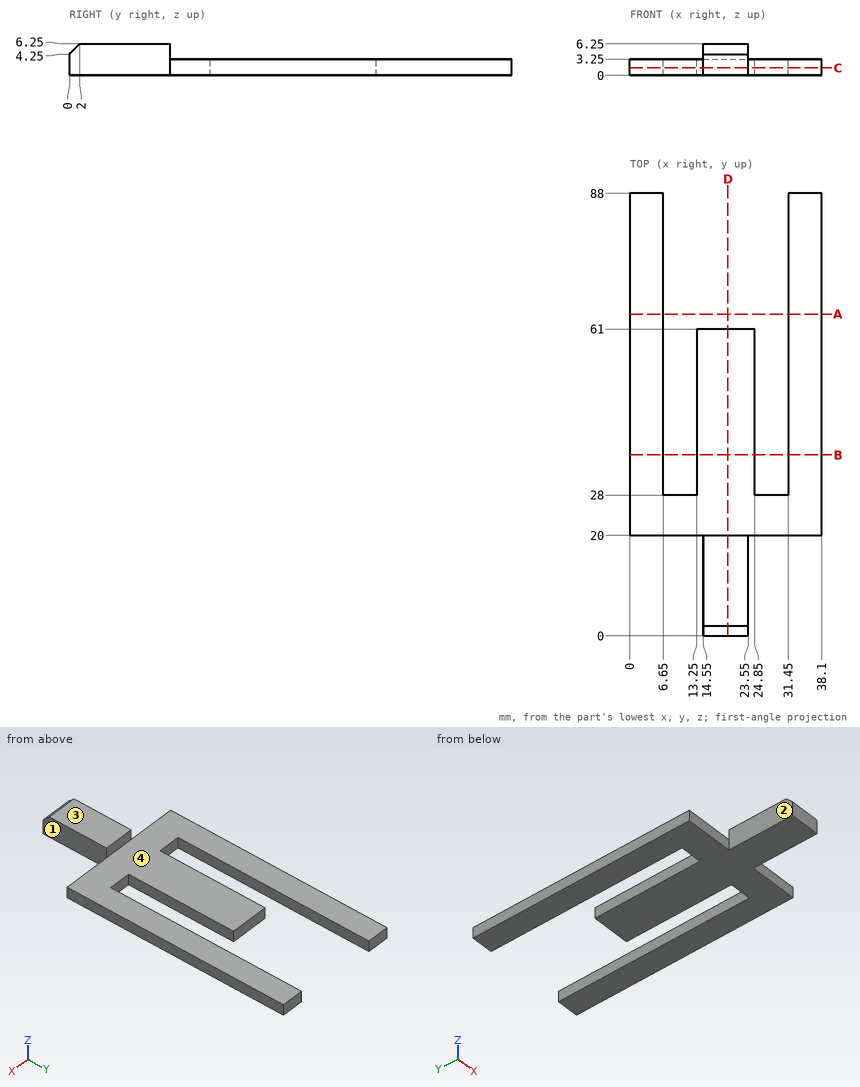
Geometry check sheet. Reference: drawing and pictorial views, mm from the part's lowest x, y, z. A direction names the side the tool comes from. Give positions to 0.01 mm unless a question says otherwise; leave off trailing zeros. Write each loop counter-clockwise with the first axis right and the second up, starting at its lowest first coordinate (ties: lowest second). Pieces come first, ordered by that corner, then holes.
Item 1: Access from +Z, -Z, +X, -X, +Y, -Y to the whole of each face (thin tool, end or side, straight path). Record for the marked faces 1, 2, 3 and 4.
Item 2: Scan lines: L1, parallel to X at y = 55, z = 1.5; L2, parallel to X at y = 79, z = 2.75; L3, parallel to Z at x = 35.5, y = 73. Record each from-to range of solid material in increasing order.
Item 3: Cross-section at A-A (y = 64). Enter the section's corners in (x, z).
Item 4: Gauge pin test, flat ends, axial feed: pin 1 (2.5 mm diameter, centred on y = 44, z = 1.5, fed in from -X); pin 2 (1 mm diameter, centred on x = 17.5, z = 5, fed in from -Y); pin 3 (19 mm diameter, centred on x = 13, y = 53, fed in from +Z); pin 4 (2.5 mm diameter, centred on x = 27.5, z = 2, fed in from +Y). Record the tip position at first contact, or that the pin passes through.
Item 5: Cross-section at D-D (x = 19.5). Enter the section's corners in (y, z), and give its area (3 significant figures).
Item 6: Cross-section at C-C (z = 1.5). Enter the section's corners in (x, y), and give its area (3 significant figures).
Item 7: Cross-section at B-B (y = 36). Enter the section's corners in (x, z), and give its area (3 significant figures).
Report:
1. face 1: +Z, -Z, +X, -Y
1. face 2: +Z, -Z, -X, -Y
1. face 3: +Z, +X, -X, +Y, -Y
1. face 4: +Z, +X, -X, +Y
2. L1: x = 0 to 6.65, 13.25 to 24.85, 31.45 to 38.1
2. L2: x = 0 to 6.65, 31.45 to 38.1
2. L3: z = 0 to 3.25
3. outline: (0, 0) - (6.65, 0) - (6.65, 3.25) - (0, 3.25) - close; (31.45, 0) - (38.1, 0) - (38.1, 3.25) - (31.45, 3.25) - close
4. pin 1: stops at x = 0
4. pin 2: stops at y = 0.25
4. pin 3: stops at z = 3.25
4. pin 4: stops at y = 28
5. outline: (0, 0) - (61, 0) - (61, 3.25) - (20, 3.25) - (20, 6.25) - (2, 6.25) - (0, 4.25) - close
5. area: 256 mm2
6. outline: (0, 20) - (14.55, 20) - (14.55, 0) - (23.55, 0) - (23.55, 20) - (38.1, 20) - (38.1, 88) - (31.45, 88) - (31.45, 28) - (24.85, 28) - (24.85, 61) - (13.25, 61) - (13.25, 28) - (6.65, 28) - (6.65, 88) - (0, 88) - close
6. area: 1,670 mm2
7. outline: (0, 0) - (6.65, 0) - (6.65, 3.25) - (0, 3.25) - close; (13.25, 0) - (24.85, 0) - (24.85, 3.25) - (13.25, 3.25) - close; (31.45, 0) - (38.1, 0) - (38.1, 3.25) - (31.45, 3.25) - close
7. area: 80.9 mm2
